The model under review builds one solid part; all positions refer to its coordinate system, in mm. A direction names the side the tool comes from. Coordinates: 2 decimals unless noted, no trailing zeros. Loops run counter-clockwise (first coordinate to the right, second up) from the corner with the lowest first, then second, coordinate; pieces in that order, holes last. Notation, with made-up numbers: M -16.5,43 L 14.5,43 A11 cw 14.5,51 Z; hole C 37.5,-36 d7. An arc over 180 degrees is marked long. Use one line per item in the form item = value.
```python
from build123d import *

# Parameters (mm, degrees)
F1_DEPTH  = 63.5
F0_W      = 30.8390699949
F0_H      = 19.05
F2_DEPTH  = 50.8
F3_DEPTH  = 15.875
F2_FACE_W = 50.8
F2_FACE_H = 19.05
F5_R      = 6.35


with BuildPart() as f1:
    # F0 (on Front) → F1 (new body, symmetric)
    with BuildSketch(Plane.XZ):
        Polygon((-41.275, -9.525), (41.275, -9.525), (41.275, 9.525), (22.225, 9.525), (-41.275, 9.525), align=None)
    extrude(amount=F1_DEPTH, both=True)

    # F0 (on Front) → F2 (join)
    with BuildSketch(Plane.XZ):
        with BuildLine():
            Line((22.225, 9.525), (41.275, 9.525))
            Line((41.275, 9.525), (41.275, 27.0002))
            ThreePointArc((41.275, 27.0002), (45.9246798487, 38.2255201513), (57.15, 42.8752))
            Line((57.15, 42.8752), (60.325, 42.8752))
            Line((60.325, 42.8752), (60.325, 61.9252))
            Line((60.325, 61.9252), (57.15, 61.9252))
            add(Edge.make_bspline(
                [(56.931387773, 61.9245157942), (57.0043014085, 61.9247938366), (57.0771722736, 61.9250219014), (57.15, 61.9252)],
                knots=[111.311302115, 111.311302115, 111.311302115, 111.311302115, 111.5045361635, 111.5045361635, 111.5045361635, 111.5045361635], degree=3))
            ThreePointArc((56.931387773, 61.9245157942), (32.3771251463, 51.6184919084), (22.225, 27.0002))
            Line((22.225, 27.0002), (22.225, 9.525))
        make_face()
        with Locations((75.7445349974, 52.4002)):
            Rectangle(F0_W, F0_H)
    extrude(amount=F2_DEPTH)

    # F0 (on Front) → F3 (join)
    with BuildSketch(Plane.XZ):
        with BuildLine():
            add(Edge.make_bspline(
                [(-41.275, 9.525), (-41.2639124943, 45.0202943965), (14.9299300749, 61.764351157), (56.931387773, 61.9245157942)],
                knots=[0, 0, 0, 0, 111.311302115, 111.311302115, 111.311302115, 111.311302115], degree=3))
            Line((-41.275, 9.525), (22.225, 9.525))
            Line((22.225, 9.525), (22.225, 27.0002))
            ThreePointArc((22.225, 27.0002), (32.3771251463, 51.6184919084), (56.931387773, 61.9245157942))
        make_face()
    extrude(amount=F3_DEPTH)

    # F0 (on Front) + F2_face (on face) → F4 (revolve)
    with BuildSketch(Plane.XZ):
        Polygon((91.1640699949, 61.9252), (91.1640699949, 42.8752), (91.1640699949, 38.1), (111.125, 38.1), (111.125, 66.675), (91.1640699949, 66.675), align=None)
    with BuildSketch(Plane(origin=(91.1640699949, -25.4, 52.4002), x_dir=(0, 1, 0), z_dir=(1, 0, 0))):
        Rectangle(F2_FACE_W, F2_FACE_H)
    revolve(axis=Axis((91.1640699949, 0, 52.3875), (0, 0, 1)))

    # F5
    f5_edges = [f1.edges().sort_by_distance(p)[0] for p in [
        (41.275, -63.5, 0),
        (-41.275, -63.5, 0),
        (-41.275, 31.75, 9.525),
        (41.275, 63.5, 0),
    ]]
    fillet(f5_edges, radius=F5_R)


solid = f1.part
```
1. Insertion check: P1, Ø8.5, axis at y = -35, z = 16, coming from the -X side (3 decimals); P2, Ø6, axis at y = 3.5, z = 52.5, coming from the +X side; P3, Ø15.5, axis at x = 41, z = 39.5, coming from the -Y side; P4, Ø6, axis at y = -9.5, z = 10.5, coming from the -X side (3 decimals). Each pin has a flat end and moves straight along its axis. Give the tip position at first contact, or say it passes through.
Response values:
P1 = 22.225
P2 = 141.96
P3 = -50.8
P4 = -41.275
2. The part is to be moulded in two halves that separate along X. For faces 1 (the face through (-39.46, 32.19, 7.62)), 2 (the face through (-9, -40, 9.525)), 3 (the face through (109.6, -7.65, 40.52)), 4 (the face through (39.464, 61.59, 0.133)), say which applies: pulls with the +X half, pulls with the -X half, needs draft (parallel to the pull), parting line crosses it, or undercut.
Response values:
face_1 = pulls with the -X half
face_2 = needs draft
face_3 = undercut
face_4 = pulls with the +X half
3. Machinability: for faces 5 (the face through (49, -50.8, 42)), 6 (the face through (45.8, -25, 38.1)), 7 (the face through (91, 0, 38.1)), 8 (the face through (1, -15.875, 30)), 9 (the face through (109.6, -7.65, 64.33)), which of the approach directions +Z, -Z, +X, -X, +Y, -Y give a long, thin tool a straight path to every point of the face, cutting with its end or side? Answer none if there is none.
Response values:
face_5 = +Z, +X, -X, -Y
face_6 = -Z, +Y, -Y
face_7 = -Z, +X, +Y, -Y
face_8 = +Z, -X, -Y
face_9 = +Z
4. Wall thickness on line 1 along Y through (x, z) = (17, 43) (3 decimals); line 2 along X through (y, z) = (-27.5, 5.5) (3 decimals); line 3 along Z through (x, y) = (-20, 14) (3 decimals): over which ranges is each line inside the solid? List them lowest first. Write a range as from..to.
Response values:
line_1 = -15.875..0
line_2 = -41.275..41.275
line_3 = -9.525..9.525
5. Add section C-C (y = 53). State the section outline as (x, z) points (3 decimals).
Response values:
outline = M -41.275,-9.525 L 41.275,-9.525 L 41.275,9.525 L -34.925,9.525 A6.35 ccw -41.275,3.175 Z
6. Add section B-B (z = -3). State the section outline as (x, y) points (3 decimals).
Response values:
outline = M -41.275,-57.15 A6.35 ccw -34.925,-63.5 L 34.925,-63.5 A6.35 ccw 41.275,-57.15 L 41.275,57.15 A6.35 ccw 34.925,63.5 L -41.275,63.5 Z
7. Add section A-A (y = 33). State the section outline as (x, z) points (3 decimals), then the cut area to 3 significant figures.
Response values:
outline = M -41.275,-9.525 L 41.275,-9.525 L 41.275,9.525 L -34.925,9.525 A6.35 ccw -41.275,3.175 Z; M 52.542,42.875 L 129.786,42.875 L 129.786,61.925 L 52.542,61.925 Z
area = 3,040 mm^2
8. Add section D-D (x = 45). State the section outline as (y, z) points.
Response values:
outline = M -50.8,37.22 L 0,37.22 L 0,42.88 L 21.2,42.88 L 21.2,61.93 L -21.2,61.93 L -21.2,59.74 L -50.8,59.74 Z
